Source: CAD feature listing. Evaluate the final solid. Frame: model axes, mm. Face numbers are marked on the shaded views. A direction names the side the tool comes from. Round coordinates to 2 decimals unless told otherwise and drop trailing zeros. Write each loop counter-clockwise with the first axis right and the second up, starting at its lowest first coordinate (ties: lowest second). Pieces come first, ordered by that corner, then holes. Notation, with made-up numbers: (19, 50.25) - (56, 50.25) arc R24 cw to (56, 80.25) - close; hole circle Ø2 at (15, 69.5). An arc over 180 degrees is marked (long way). Write item = value, one per line. Start each with the question number.
```python
from build123d import *

# Parameters (mm, degrees)
EXTRUDE_1_DEPTH          = 110
CUT_EXTRUDE_1_REACH      = 180.332
SKETCH_2_R               = 31.5
PATTERN_CIRCULAR_1_COUNT = 4
PATTERN_CIRCULAR_1_ANGLE = 90


with BuildPart() as part:
    # 草图1 → 凸台-拉伸1 (new body)
    with BuildSketch(Plane.XY):
        Polygon((-100, -17.5), (-62.5, -17.5), (-62.5, -98.5), (62.5, -98.5), (62.5, -17.5), (100, -17.5), (100, 17.5), (-100, 17.5), align=None)
    extrude(amount=EXTRUDE_1_DEPTH)

    # 草图2 → 切除-拉伸1 (cut, up to next)
    with BuildSketch(Plane(origin=(0, 0, 0), x_dir=(-1, 0, 0), z_dir=(0, 0, -1)), mode=Mode.PRIVATE) as cut_extrude_1_sk1:
        with Locations((0, -43)):
            Circle(SKETCH_2_R)
    cut_extrude_1_tool1 = extrude(cut_extrude_1_sk1.sketch, amount=-CUT_EXTRUDE_1_REACH, mode=Mode.PRIVATE) & part.part
    add(cut_extrude_1_tool1.solids().sort_by_distance((0, -43, 0))[0], mode=Mode.SUBTRACT)

    # 草图5 → M10 螺纹孔1 (revolve, cut)
    with BuildSketch(Plane(origin=(-32.88, -10.119069356, 0), x_dir=(0, 1, 0), z_dir=(1, 0, 0))):
        Polygon((0, 0), (0, 30), (4.25, 27.446342369), (4.25, 0), align=None)
    hole_wizard_m10_1 = revolve(axis=Axis((-32.88, -10.119069356, -6.35), (0, 0, 1)), mode=Mode.SUBTRACT)

    # 阵列(圆周)1: M10 螺纹孔1 ×4 about axis
    pattern_circular_1_axis = Axis((0, -43, 0), (0, 0, 1))
    for i in range(1, PATTERN_CIRCULAR_1_COUNT):
        add(hole_wizard_m10_1.rotate(pattern_circular_1_axis, i * PATTERN_CIRCULAR_1_ANGLE / (PATTERN_CIRCULAR_1_COUNT - 1)), mode=Mode.SUBTRACT)

    # 镜向1: M10 螺纹孔1 across plane
    add(hole_wizard_m10_1.mirror(Plane(origin=(0, 0, 0), x_dir=(0, 0, 1), z_dir=(1, 0, 0))), mode=Mode.SUBTRACT)

    # 镜向1 copy 1 sketch → 镜向1 copy 1 (revolve, cut)
    with BuildSketch(Plane(origin=(44.915380598, -30.964278762, 0), x_dir=(0.5000000000000011, 0.866025403784438, 0), z_dir=(-0.866025403784438, 0.5000000000000011, 0))):
        Polygon((0, 0), (0, -30), (4.25, -27.446342369), (4.25, 0), align=None)
    revolve(axis=Axis((44.915380598, -30.964278762, -6.35), (0, 0, -1)), mode=Mode.SUBTRACT)

    # 镜向1 copy 2 sketch → 镜向1 copy 2 (revolve, cut)
    with BuildSketch(Plane(origin=(44.915721238, -55.034449955, 0), x_dir=(0.8660254037844399, 0.4999999999999978, 0), z_dir=(-0.4999999999999978, 0.8660254037844399, 0))):
        Polygon((0, 0), (0, -30), (4.25, -27.446342369), (4.25, 0), align=None)
    revolve(axis=Axis((44.915721238, -55.034449955, -6.35), (0, 0, -1)), mode=Mode.SUBTRACT)

    # 镜向1 copy 3 sketch → 镜向1 copy 3 (revolve, cut)
    with BuildSketch(Plane(origin=(32.880930644, -75.88, 0), x_dir=(1, 0, 0), z_dir=(0, 1, 0))):
        Polygon((0, 0), (0, -30), (4.25, -27.446342369), (4.25, 0), align=None)
    revolve(axis=Axis((32.880930644, -75.88, -6.35), (0, 0, -1)), mode=Mode.SUBTRACT)


solid = part.part
```
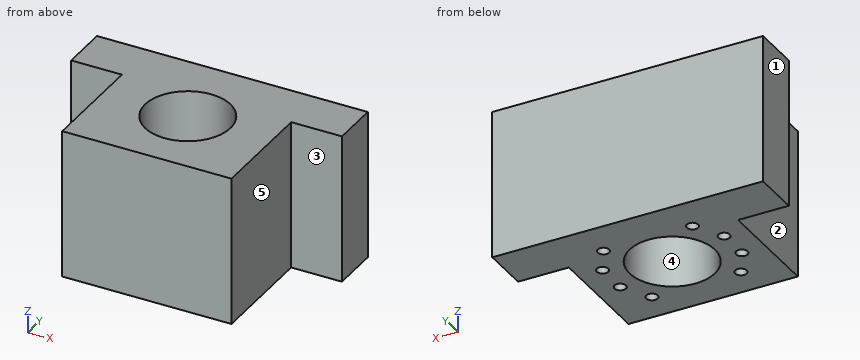
(1) Ray query, L1, parallel to X at y = -75.88, z = 9; L2, parallel to X at y = -52, z = 14.5; L3, parallel to Y at x = -42, z = 15.5. Return the intervals inside material, ascending. Write a range as from..to.
(2) Section D-D (z = 24). Count the separate pieces of the cut face and the enclosed holes in it, plus the area to 3 significant figures.
(3) Reachability of the marked faces 1 and 2 from +Z, -Z, +X, -X, +Y, -Y: full face, straight path, thin tool, end or side. Return the list, or none.
(4) Contact query for flat-ended pins moving along their axis: P1, Ø10, axis at x = -44.92, y = -55.03, coming from the -Z side; P2, Ø2, axis at x = 69.5, z = 87.5, coming from the -Y side; P3, Ø7.5, axis at x = -44.92, y = -30.96, coming from the -Z side; P4, Ø12, axis at y = -83, z = 37.5, coming from the -X side. Output: stop coordinate, or through.
(5) Section A-A (y = -43). Return the cut outline in (x, z), plus the area to 3 significant figures.
(6) Section B-B (x = 0). Return the cut outline in (y, z).
(7) Pull-direction query (Y, two-part tool) for the marked faces 3, 4 and 5; classes: +Y half, -Y half, draft (parallel to the pull), parting line (faces both ways), or undercut.
(8) Section C-C (z = 41.5). Return the cut outline in (x, y), plus the area to 3 significant figures.
Solution:
q1.L1 = -62.5..-37.13, -28.63..28.63, 37.13..62.5
q1.L2 = -62.5..-47.89, -41.94..-30.19, 30.19..41.94, 47.89..62.5
q1.L3 = -98.5..-58.13, -51.94..-34.06, -27.87..17.5
q2.separate_pieces = 1
q2.enclosed_holes = 9
q2.area = 13,600 mm^2
q3.face_1 = +Z, -Z, -X, +Y, -Y
q3.face_2 = +Z, -Z, -X, -Y
q4.P1 = 0
q4.P2 = -17.5
q4.P3 = 27.74
q4.P4 = -62.5
q5.outline = (-62.5, 0) - (-31.5, 0) - (-31.5, 110) - (-62.5, 110) - close; (31.5, 0) - (62.5, 0) - (62.5, 110) - (31.5, 110) - close
q5.area = 6,820 mm^2
q6.outline = (-98.5, 0) - (-74.5, 0) - (-74.5, 110) - (-98.5, 110) - close; (-11.5, 0) - (17.5, 0) - (17.5, 110) - (-11.5, 110) - close
q7.face_3 = -Y half
q7.face_4 = undercut
q7.face_5 = draft
q8.outline = (-100, -17.5) - (-62.5, -17.5) - (-62.5, -98.5) - (62.5, -98.5) - (62.5, -17.5) - (100, -17.5) - (100, 17.5) - (-100, 17.5) - close; hole circle Ø63 at (0, -43)
q8.area = 14,000 mm^2
